Verification items for the finished model (mm, model axes). Give positions to 0.01 mm unless a question says otherwise; leave off trailing zeros. Write each loop counter-clockwise with the first axis right and the second up, starting at its lowest first coordinate (ties: lowest second). Pieces come first, ordered by that corner, then holes.
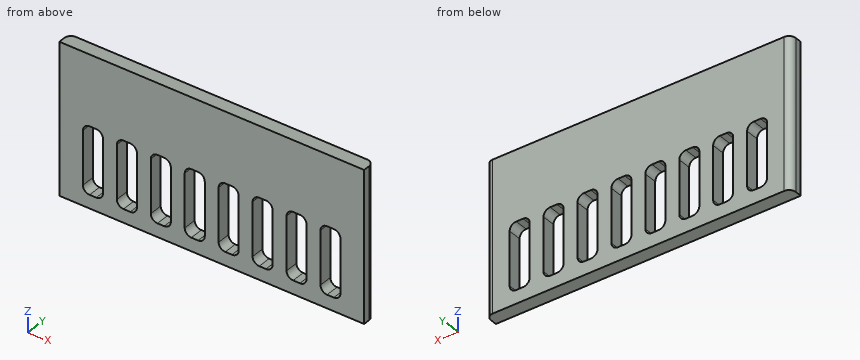
from build123d import *

# Parameters (mm, degrees)
BOX036_W     = 3
BOX036_H     = 10.16
BOX036_DEPTH = 10
FILLET002_R  = 1
BOX035_W     = 3
BOX035_H     = 10.16
BOX035_DEPTH = 10
FILLET001_R  = 1
BOX037_W     = 3
BOX037_H     = 10.16
BOX037_DEPTH = 10
FILLET003_R  = 1
BOX038_W     = 3
BOX038_H     = 10.16
BOX038_DEPTH = 10
FILLET004_R  = 1
BOX039_W     = 3
BOX039_H     = 10.16
BOX039_DEPTH = 10
FILLET005_R  = 1
BOX040_W     = 3
BOX040_H     = 10.16
BOX040_DEPTH = 10
FILLET006_R  = 1
BOX041_W     = 3
BOX041_H     = 10.16
BOX041_DEPTH = 10
FILLET007_R  = 1
BOX032_W     = 3
BOX032_H     = 10.16
BOX032_DEPTH = 10
FILLET_R     = 1
BOX021_W     = 45.64
BOX021_H     = 2
BOX021_DEPTH = 22.5
FILLET008_R  = 1


with BuildPart() as fillet002:
    # Box036 → Box036 (new body)
    with BuildSketch(Plane(origin=(49.3, 45.775, 2), x_dir=(1, 0, 0), z_dir=(0, 0, 1))):
        with Locations((1.5, 5.08)):
            Rectangle(BOX036_W, BOX036_H)
    extrude(amount=BOX036_DEPTH)

    # Fillet002
    fillet002_edges = [fillet002.edges().sort_by_distance(p)[0] for p in [
        (49.3, 50.855, 12),
        (49.3, 50.855, 2),
        (52.3, 50.855, 12),
        (52.3, 50.855, 2),
    ]]
    fillet(fillet002_edges, radius=FILLET002_R)


with BuildPart() as fillet001:
    # Box035 → Box035 (new body)
    with BuildSketch(Plane(origin=(54.38, 45.775, 2), x_dir=(1, 0, 0), z_dir=(0, 0, 1))):
        with Locations((1.5, 5.08)):
            Rectangle(BOX035_W, BOX035_H)
    extrude(amount=BOX035_DEPTH)

    # Fillet001
    fillet001_edges = [fillet001.edges().sort_by_distance(p)[0] for p in [
        (54.38, 50.855, 12),
        (54.38, 50.855, 2),
        (57.38, 50.855, 12),
        (57.38, 50.855, 2),
    ]]
    fillet(fillet001_edges, radius=FILLET001_R)


with BuildPart() as fillet003:
    # Box037 → Box037 (new body)
    with BuildSketch(Plane(origin=(44.22, 45.775, 2), x_dir=(1, 0, 0), z_dir=(0, 0, 1))):
        with Locations((1.5, 5.08)):
            Rectangle(BOX037_W, BOX037_H)
    extrude(amount=BOX037_DEPTH)

    # Fillet003
    fillet003_edges = [fillet003.edges().sort_by_distance(p)[0] for p in [
        (44.22, 50.855, 12),
        (44.22, 50.855, 2),
        (47.22, 50.855, 12),
        (47.22, 50.855, 2),
    ]]
    fillet(fillet003_edges, radius=FILLET003_R)


with BuildPart() as fillet004:
    # Box038 → Box038 (new body)
    with BuildSketch(Plane(origin=(39.14, 45.775, 2), x_dir=(1, 0, 0), z_dir=(0, 0, 1))):
        with Locations((1.5, 5.08)):
            Rectangle(BOX038_W, BOX038_H)
    extrude(amount=BOX038_DEPTH)

    # Fillet004
    fillet004_edges = [fillet004.edges().sort_by_distance(p)[0] for p in [
        (39.14, 50.855, 12),
        (39.14, 50.855, 2),
        (42.14, 50.855, 12),
        (42.14, 50.855, 2),
    ]]
    fillet(fillet004_edges, radius=FILLET004_R)


with BuildPart() as fillet005:
    # Box039 → Box039 (new body)
    with BuildSketch(Plane(origin=(34.06, 45.775, 2), x_dir=(1, 0, 0), z_dir=(0, 0, 1))):
        with Locations((1.5, 5.08)):
            Rectangle(BOX039_W, BOX039_H)
    extrude(amount=BOX039_DEPTH)

    # Fillet005
    fillet005_edges = [fillet005.edges().sort_by_distance(p)[0] for p in [
        (34.06, 50.855, 12),
        (34.06, 50.855, 2),
        (37.06, 50.855, 12),
        (37.06, 50.855, 2),
    ]]
    fillet(fillet005_edges, radius=FILLET005_R)


with BuildPart() as fillet006:
    # Box040 → Box040 (new body)
    with BuildSketch(Plane(origin=(28.98, 45.775, 2), x_dir=(1, 0, 0), z_dir=(0, 0, 1))):
        with Locations((1.5, 5.08)):
            Rectangle(BOX040_W, BOX040_H)
    extrude(amount=BOX040_DEPTH)

    # Fillet006
    fillet006_edges = [fillet006.edges().sort_by_distance(p)[0] for p in [
        (28.98, 50.855, 12),
        (28.98, 50.855, 2),
        (31.98, 50.855, 12),
        (31.98, 50.855, 2),
    ]]
    fillet(fillet006_edges, radius=FILLET006_R)


with BuildPart() as fillet007:
    # Box041 → Box041 (new body)
    with BuildSketch(Plane(origin=(23.9, 45.775, 2), x_dir=(1, 0, 0), z_dir=(0, 0, 1))):
        with Locations((1.5, 5.08)):
            Rectangle(BOX041_W, BOX041_H)
    extrude(amount=BOX041_DEPTH)

    # Fillet007
    fillet007_edges = [fillet007.edges().sort_by_distance(p)[0] for p in [
        (23.9, 50.855, 12),
        (23.9, 50.855, 2),
        (26.9, 50.855, 12),
        (26.9, 50.855, 2),
    ]]
    fillet(fillet007_edges, radius=FILLET007_R)


with BuildPart() as fusion:
    # Box032 → Box032 (new body)
    with BuildSketch(Plane(origin=(59.46, 45.775, 2), x_dir=(1, 0, 0), z_dir=(0, 0, 1))):
        with Locations((1.5, 5.08)):
            Rectangle(BOX032_W, BOX032_H)
    extrude(amount=BOX032_DEPTH)

    # Fillet
    fillet_edges = [fusion.edges().sort_by_distance(p)[0] for p in [
        (59.46, 50.855, 12),
        (59.46, 50.855, 2),
        (62.46, 50.855, 12),
        (62.46, 50.855, 2),
    ]]
    fillet(fillet_edges, radius=FILLET_R)

    # Fusion: union Fillet002, Fillet001, Fillet003, Fillet004, Fillet005, Fillet006, Fillet007
    add(fillet002.part)
    add(fillet001.part)
    add(fillet003.part)
    add(fillet004.part)
    add(fillet005.part)
    add(fillet006.part)
    add(fillet007.part)


with BuildPart() as cut:
    # Box021 → Box021 (new body)
    with BuildSketch(Plane(origin=(20.36, 51.935, 0), x_dir=(1, 0, 0), z_dir=(0, 0, 1))):
        with Locations((22.82, 1)):
            Rectangle(BOX021_W, BOX021_H)
    extrude(amount=BOX021_DEPTH)

    # Fillet008
    fillet008_edges = [cut.edges().sort_by_distance(p)[0] for p in [
        (20.36, 53.935, 11.25),
        (66, 53.935, 11.25),
    ]]
    fillet(fillet008_edges, radius=FILLET008_R)

    # Cut: cut Fusion
    add(fusion.part, mode=Mode.SUBTRACT)


solid = cut.part
Item 1: Depth check by flat-ended pin: pin 1 (1.1 mm diameter, centred on x = 50.5, y = 53, fed in from -Z). Enter the tip coordinate at first touch or a pass-through.
Answer key:
pin 1: stops at z = 0
Item 2: Sectioned sample at A-A on x = 61. Record the cut outline in (y, z) (3 decimals).
Answer key:
outline: (51.935, 0) - (53.935, 0) - (53.935, 2) - (51.935, 2) - close; (51.935, 12) - (53.935, 12) - (53.935, 22.5) - (51.935, 22.5) - close
Item 3: Sectioned sample at B-B on z = 3.5. State how many separate pieces and enclosed holes the cut face has, then the cut area to 3 significant figures.
Answer key:
separate pieces: 9
enclosed holes: 0
area: 42.9 mm2
Item 4: Scan lines: line 1 along Z through (x, y) = (31, 53.7); line 2 along Z through (x, y) = (44.5, 52.45); line 3 along X through (y, z) = (53.4, 16.5). Record each from-to range of solid material in increasing order.
Answer key:
line 1: z = 0 to 2, 12 to 22.5
line 2: z = 0 to 2.31, 11.69 to 22.5
line 3: x = 20.47 to 65.89
